Check sheet for the drawn part. Datum: minimum x, y, z corner. Units: mm. Coordinates: 2 decimals unless noted, no trailing zeros. Loops run counter-clockwise (first coordinate to the right, second up) from the corner with the lowest first, then second, coordinate; pieces in that order, holes last.
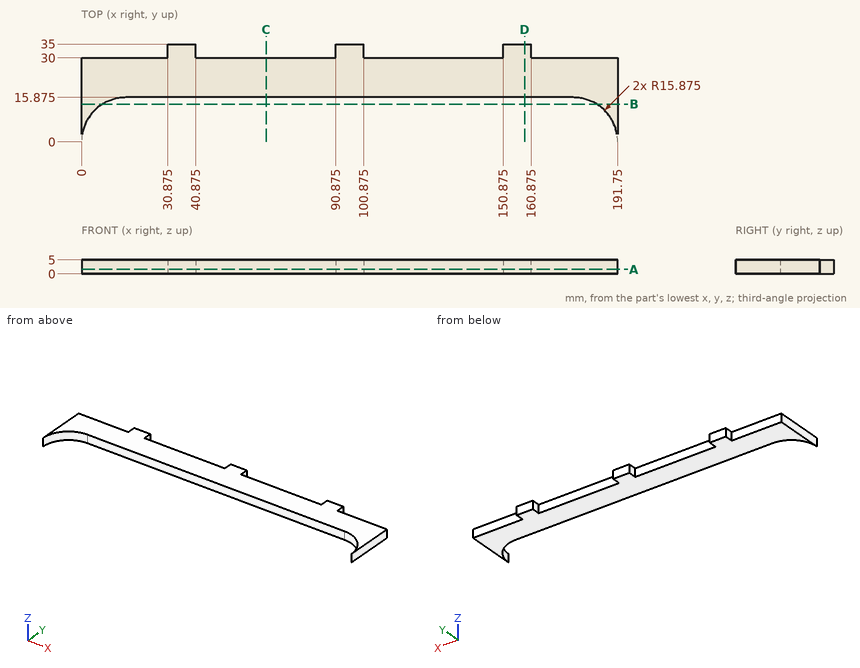
1) Scan lines: line 1 (X direction, y = 33, z = 4.05) (3 decimals); line 2 (Y direction, x = 44, z = 2.85) (3 decimals); line 3 (Y direction, x = 99, z = 2.2) (3 decimals). Record each from-to range of solid material in increasing order.
Answer sheet:
line 1: x = 30.875 to 40.875, 90.875 to 100.875, 150.875 to 160.875
line 2: y = 15.875 to 30
line 3: y = 15.875 to 35
2) Section check B-B on y = 13.5. Enter the section's corners in (x, z).
Answer sheet:
outline: (0, 0) - (7.52, 0) - (7.52, 5) - (0, 5) - close; (184.23, 0) - (191.75, 0) - (191.75, 5) - (184.23, 5) - close
3) Section check D-D on x = 158.5. Enter the section's corners in (y, z) (3 decimals), plus the area to 3 significant figures.
Answer sheet:
outline: (15.875, 0) - (35, 0) - (35, 5) - (15.875, 5) - close
area: 95.6 mm2
4) Depth check by flat-ended pin: pin 1 (2.5 mm diameter, centred on x = 176, z = 3.5, fed in from +Y); pin 2 (2.5 mm diameter, centred on y = 31.5, z = 3, fed in from -X) (3 decimals); pin 3 (2.5 mm diameter, centred on y = 32, z = 3.5, fed in from +X) (3 decimals); pin 4 (12 mm diameter, centred on x = 82.5, y = 4.5, fed in from +Z). Enter the tip coordinate at first touch or a pass-through.
Answer sheet:
pin 1: stops at y = 30
pin 2: stops at x = 30.875
pin 3: stops at x = 160.875
pin 4: passes through
5) Section check A-A on z = 1.6. Enter the section's corners in (x, y) (3 decimals).
Answer sheet:
outline: (0, 0) arc R15.875 cw to (15.875, 15.875) - (175.875, 15.875) arc R15.875 cw to (191.75, 0) - (191.75, 30) - (160.875, 30) - (160.875, 35) - (150.875, 35) - (150.875, 30) - (100.875, 30) - (100.875, 35) - (90.875, 35) - (90.875, 30) - (40.875, 30) - (40.875, 35) - (30.875, 35) - (30.875, 30) - (0, 30) - close
6) Section check C-C on x = 66. Enter the section's corners in (y, z) (3 decimals), plus the area to 3 significant figures.
Answer sheet:
outline: (15.875, 0) - (30, 0) - (30, 5) - (15.875, 5) - close
area: 70.6 mm2
